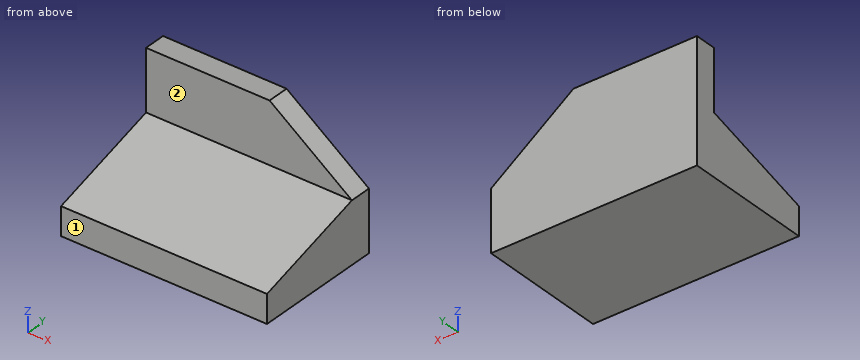
```python
from build123d import *

# Parameters (mm, degrees)
F1_DEPTH = 95
F3_DEPTH = 25


with BuildPart() as f1:
    # F0 (on Right) → F1 (new body)
    with BuildSketch(Plane.YZ):
        Polygon((-60, 0), (0, 0), (0, 56), (-10, 56), (-10, 28), (-60, 13), align=None)
    extrude(amount=F1_DEPTH)

    # F2 (on face) → F3 (cut)
    with BuildSketch(Plane.XZ.offset(10)):
        Polygon((95, 56), (57, 56), (95, 28), align=None)
    extrude(amount=-F3_DEPTH, mode=Mode.SUBTRACT)


solid = f1.part
```
Input: part model. Units: mm. Frame: model coordinates. Face numbers are marked on the shaded views. A direction names the side the tool comes from. Give positions to 0.01 mm unless a question says otherwise; leave off trailing zeros. Order: outer loops, then holes, each group sorted by start corner. A loop starts at its lowest first (then second) coordinate and runs counter-clockwise, first axis right, second up. Notation, with made-up numbers: M 25.25,34.5 L 79.25,34.5 A25 cw 79.25,68.5 Z; hole C 57,87 d8. An arc over 180 degrees is marked long. Return JSON: item names as keys, results as strings.
Item 1: Ray query, probe 1 along Y at (x, z) = (45, 42); probe 2 along Z at (x, y) = (89.5, -55.5); probe 3 along Z at (x, y) = (73, -49.5). Return the intervals inside material, ascending.
Solutions:
{"probe 1": "-10 to 0", "probe 2": "0 to 14.35", "probe 3": "0 to 16.15"}
Item 2: Cut plane B-B (y = -44.5). Return loops of the section in (x, z), then the cut area to 3 significant figures.
Solutions:
{"outline": "M 0,0 L 95,0 L 95,17.65 L 0,17.65 Z", "area": "1,680 mm^2"}
Item 3: First-contact query: P1, Ø1.5, axis at x = 24.5, z = 46.5, coming from the -Y side. Flat tip, straight axial feed; report the tip coordinate or a pass-through.
Solutions:
{"P1": "y = -10"}
Item 4: Access query for the marked faces 1 and 2. Directions: +Z, -Z, +X, -X, +Y, -Y. A direction counts if a zero-diameter tool reaches every point of the face in a straight line with its end or side. Return the directions, or none.
Solutions:
{"face 1": "+Z, -Z, +X, -X, -Y", "face 2": "+Z, +X, -X, -Y"}
Item 5: Cut plane A-A (x = 51). Return loops of the section in (y, z).
Solutions:
{"outline": "M -60,0 L 0,0 L 0,56 L -10,56 L -10,28 L -60,13 Z"}
Item 6: Cut plane C-C (z = 31.5). Return loops of the section in (x, y), then the cut area to 4 significant figures.
Solutions:
{"outline": "M 0,-10 L 90.25,-10 L 90.25,0 L 0,0 Z", "area": "902.5 mm^2"}
